Could you check a few things on this model? Use its own coordinates, in mm. A direction names the side the tool comes from. Coordinates: 2 decimals unless noted, no trailing zeros. Loops run counter-clockwise (first coordinate to the right, second up) from the corner with the lowest first, then second, coordinate; pieces in that order, holes last.
from build123d import *

# Parameters (mm, degrees)
F0_R     = 9.525
F1_DEPTH = 25.4
F3_DEPTH = 25.401
F4_DEPTH = 12.7
F6_DEPTH = 9.525


with BuildPart() as f1:
    # F0 (on Front) → F1 (new body)
    with BuildSketch(Plane.XZ):
        Circle(F0_R)
    extrude(amount=F1_DEPTH)

    # F2 (on face) → F3 (cut, through all)
    with BuildSketch(Plane(origin=(0, 0, 0), x_dir=(-1, 0, 0), z_dir=(0, 1, 0))):
        with BuildLine():
            ThreePointArc((-4.7625, 0), (-3.367596, -3.367596), (0, -4.7625))
            ThreePointArc((0, -4.7625), (3.367596, -3.367596), (4.7625, 0))
            ThreePointArc((4.7625, 0), (3.367596, 3.367596), (0, 4.7625))
            ThreePointArc((0, 4.7625), (-3.367596, 3.367596), (-4.7625, 0))
        make_face()
    extrude(amount=-F3_DEPTH, mode=Mode.SUBTRACT)

    # F2 (on face) → F4 (cut)
    with BuildSketch(Plane(origin=(0, 0, 0), x_dir=(-1, 0, 0), z_dir=(0, 1, 0))):
        with BuildLine():
            Line((-4.7625, 0), (-4.7625, -4.7625))
            Line((-4.7625, -4.7625), (0, -4.7625))
            ThreePointArc((0, -4.7625), (-3.367596, -3.367596), (-4.7625, 0))
        make_face()
        with BuildLine():
            ThreePointArc((4.7625, 0), (3.367596, -3.367596), (0, -4.7625))
            Line((0, -4.7625), (4.7625, -4.7625))
            Line((4.7625, -4.7625), (4.7625, 0))
        make_face()
        with BuildLine():
            Line((-4.7625, 4.7625), (-4.7625, 0))
            ThreePointArc((-4.7625, 0), (-3.367596, 3.367596), (0, 4.7625))
            Line((0, 4.7625), (-4.7625, 4.7625))
        make_face()
        with BuildLine():
            ThreePointArc((0, 4.7625), (3.367596, 3.367596), (4.7625, 0))
            Line((4.7625, 0), (4.7625, 4.7625))
            Line((4.7625, 4.7625), (0, 4.7625))
        make_face()
    extrude(amount=-F4_DEPTH, mode=Mode.SUBTRACT)

    # F5 (on face) → F6 (cut)
    with BuildSketch(Plane.XZ.offset(25.4)):
        Polygon((3.65125, 6.324151), (-3.65125, 6.324151), (-7.3025, 0), (-3.65125, -6.324151), (3.65125, -6.324151), (7.3025, 0), align=None)
    extrude(amount=-F6_DEPTH, mode=Mode.SUBTRACT)


solid = f1.part
(1) I need wall thicknesses on probe 1 along Y at (x, z) = (-6, -1.75) (3 decimals); probe 2 along X at (y, z) = (-24, -2.5); probe 3 along Y at (x, z) = (3.75, 3.5) (3 decimals). Which ranges of each line are inside material? Lowest first, please.
Answers:
probe 1: y = -15.875 to 0
probe 2: x = -9.19 to -5.86, 5.86 to 9.19
probe 3: y = -15.875 to -12.7
(2) We'd pull the mould along X, two halves only. Please class faces 4 (the face through (0, -21, 6.324)), 5 (the face through (6.2, -25.4, 2.3)), 6 (the face through (-7.559, -12.522, -5.796)): +X half, -X half, draft (parallel to the pull), parting line (faces both ways), or undercut.
Answers:
face 4: undercut
face 5: draft
face 6: parting line
(3) Which directions (+Z, -Z, +X, -X, +Y, -Y) give clear straight access to the entire face, cutting with the end or side of a thin tool? Please do faces 1 (the face through (-4, -12.7, -4)), 2 (the face through (5.5, -20.7, 3.12)), 3 (the face through (0, 0, -6)).
Answers:
face 1: +Y
face 2: -Y
face 3: +Z, -Z, +X, -X, +Y
(4) Imagine slicing it at B-B, the plane x = -2. Write out the boundary of the cut face in (y, z) (1 decimal), and give its area (3 significant figures).
Answers:
outline: (-25.4, -9.3) - (0, -9.3) - (0, -4.8) - (-12.7, -4.8) - (-12.7, -4.3) - (-15.9, -4.3) - (-15.9, -6.3) - (-25.4, -6.3) - close; (-25.4, 6.3) - (-15.9, 6.3) - (-15.9, 4.3) - (-12.7, 4.3) - (-12.7, 4.8) - (0, 4.8) - (0, 9.3) - (-25.4, 9.3) - close
area: 204 mm2
(5) Imagine slicing it at C-C, the plane z = 4.25. Write out the boundary of the cut face in (x, y) (1 decimal), and give its area (3 significant figures).
Answers:
outline: (-8.5, -25.4) - (-4.8, -25.4) - (-4.8, -15.9) - (-2.1, -15.9) - (-2.1, -12.7) - (-4.8, -12.7) - (-4.8, 0) - (-8.5, 0) - close; (2.1, -15.9) - (4.8, -15.9) - (4.8, -25.4) - (8.5, -25.4) - (8.5, 0) - (4.8, 0) - (4.8, -12.7) - (2.1, -12.7) - close
area: 206 mm2
(6) For pin 1 (4 mm diameter, centred on x = 3.5, z = 2.5, fed in from +Y); pin 2 (4 mm diameter, centred on x = -1.5, z = -2.5, fed in from +Y); pin 3 (8 mm diameter, centred on y = -21, z = 6, fed in from -X); pin 4 (1 mm diameter, centred on y = -10.5, z = 4, fed in from -X), each with a flat end and sliding along its axis, tell me the tip position at first contact or that it passes through.
Answers:
pin 1: stops at y = 0
pin 2: stops at y = -12.7
pin 3: stops at x = -9.31
pin 4: stops at x = -8.86
